Autodesk Inventor part; units mm, degrees
ref_plane "YZ Plane" through (0, 0, 0) normal (1, 0, 0) x (0, 1, 0)
ref_plane "XZ Plane" through (0, 0, 0) normal (0, 1, 0) x (-1, 0, 0)
ref_plane "XY Plane" through (0, 0, 0) normal (0, 0, 1) x (1, 0, 0)
sketch "Sketch1" plane through (0, 0, 0) normal (0, 1, 0) x (-1, 0, 0)
  line L0 (-40, -47.5) -> (40, -47.5)
  line L1 (40, -47.5) -> (40, 47.5)
  line L2 (40, 47.5) -> (-40, 47.5)
  line L3 (-40, 47.5) -> (-40, -47.5)
  line L4 (-40, -47.5) -> (40, 47.5) construction
  line L5 (40, -47.5) -> (-40, 47.5) construction
  line L6 (0, 0) -> (0, -31.5)
  line L7 (0, -31.5) -> (8.5, -31.5)
  line L8 (0, 0) -> (2.25, 0)
  line L9 (0, 0) -> (0, 17.5)
  line L10 (0, 17.5) -> (0, 19)
  line L11 (0, 19) -> (24, 19)
  line L12 (0, -17.5) -> (0, -19)
  line L13 (0, 31.5) -> (-19.5, 31.5)
  line L14 (0, 0) -> (0, 31.5)
  line L15 (0, 31.5) -> (8.5, 31.5)
  circle A0 centre (8.5, 31.5) radius 2.5
  line L16 (0, -19) -> (24, -19)
  circle A1 centre (24, -19) radius 2.5
  line L17 (0, 0) -> (0, -17.5)
  circle A2 centre (-19.5, 31.5) radius 2.5
  circle A3 centre (-19.5, 31.5) radius 2.5
  point P0 (0.5, 0.75)
  point P1 (0.5, -0.75)
  dimension "d0" = 80
  dimension "d1" = 95
  dimension "d2" = 17.5
  dimension "d3" = 8.5
  dimension "d5" = 31.5
  dimension "d6" = 24
  dimension "d7" = 2.25
  dimension "d12" = 19.5
extrude "Extrusion1" add sketch "Sketch1" along normal blind 10
sketch "Sketch2" plane through (0, 10, 0) normal (0, 1, 0) x (1, 0, 0)
  line L0 (-40, -47.5) -> (40, -47.5)
  line L1 (-40, -47.5) -> (-40, -36.5)
  line L2 (-40, 47.5) -> (-40, -47.5)
  line L3 (-40, -36.5) -> (-33.6491, -47.5)
  line L4 (-40, -36.5) -> (-27.2983, -36.5) construction
  line L5 (-33.6491, -47.5) -> (-33.6491, -43.5)
  line L6 (-40, -36.5) -> (-40, -33.5)
  line L7 (-33.6491, -47.5) -> (-33.6491, -45.5)
  line L8 (-32.6491, -47.5) -> (-31.6491, -47.5)
  line L9 (0, 0) -> (0, -47.5)
  line L10 (-40, -33.5) -> (-31, -33.5)
  line L11 (-31, -33.5) -> (-31, -47.5)
  line L12 (-33.6491, -47.5) -> (-31, -47.5)
  line L13 (40, -47.5) -> (40, -36.5)
  line L14 (40, -36.5) -> (33.6491, -47.5)
  line L15 (40, -36.5) -> (27.2983, -36.5) construction
  line L16 (33.6491, -47.5) -> (33.6491, -43.5)
  line L17 (40, -36.5) -> (40, -33.5)
  line L18 (33.6491, -47.5) -> (33.6491, -45.5)
  line L19 (32.6491, -47.5) -> (31.6491, -47.5)
  line L20 (40, -33.5) -> (31, -33.5)
  line L21 (31, -33.5) -> (31, -47.5)
  line L22 (33.6491, -47.5) -> (31, -47.5)
  line L23 (-40, 47.5) -> (-31, 47.5)
  line L24 (-31, 47.5) -> (-31, 33.5)
  line L25 (-31, 33.5) -> (-40, 33.5)
  line L26 (-40, 33.5) -> (-40, 47.5)
  line L27 (40, -47.5) -> (40, 47.5)
  line L28 (40, 47.5) -> (31, 47.5)
  line L29 (31, 47.5) -> (31, 33.5)
  line L30 (31, 33.5) -> (40, 33.5)
  line L31 (40, 33.5) -> (40, 47.5)
  dimension "d15" = 11
  dimension "d16" = 60
  dimension "d18" = 3
  dimension "d20" = 2
  dimension "d21" = 9
  dimension "d22" = 9
  dimension "d23" = 14
  dimension "d24" = 9
  dimension "d25" = 14
extrude "Extrusion2" add sketch "Sketch2" along normal blind 100 contours L2 L23 L24 L25 | L30 L29 L28 L27 | L21 L20 L17 L14 L0 | L3 L2 L10 L11 L0
sketch "Sketch4" plane through (0, 110, 0) normal (0, 1, 0) x (1, 0, 0)
  line L0 (-40, 47.5) -> (-40, 33.5)
  line L1 (-40, 33.5) -> (-31, 33.5)
  line L2 (-31, 33.5) -> (-31, 47.5)
  line L3 (-31, 47.5) -> (-40, 47.5)
  line L4 (40, 47.5) -> (31, 47.5)
  line L5 (31, 47.5) -> (31, 33.5)
  line L6 (31, 33.5) -> (40, 33.5)
  line L7 (40, 33.5) -> (40, 47.5)
  line L8 (33.6491, -47.5) -> (40, -36.5)
  line L9 (40, -36.5) -> (40, -33.5)
  line L10 (40, -33.5) -> (31, -33.5)
  line L11 (31, -33.5) -> (31, -47.5)
  line L12 (31, -47.5) -> (33.6491, -47.5)
  line L13 (-31, -47.5) -> (-31, -33.5)
  line L14 (-33.6491, -47.5) -> (-31, -47.5)
  line L15 (-31, -47.5) -> (-31, -33.5)
  line L16 (-31, -33.5) -> (-40, -33.5)
  line L17 (-40, -33.5) -> (-40, -36.5)
  line L18 (-40, -36.5) -> (-33.6491, -47.5)
  line L19 (-33.6491, -47.5) -> (-40, -36.5)
  line L20 (-40, -36.5) -> (-40, -47.5)
  line L21 (-40, -47.5) -> (-33.6491, -47.5)
  line L22 (40, -36.5) -> (33.6491, -47.5)
  line L23 (33.6491, -47.5) -> (40, -47.5)
  line L24 (40, -47.5) -> (40, -36.5)
  line L25 (-40, 47.5) -> (40, 47.5)
  line L26 (-40, 47.5) -> (-40, -47.5)
  line L27 (40, -47.5) -> (-40, -47.5)
  line L28 (-40, -47.5) -> (40, -47.5)
  line L29 (40, -47.5) -> (40, 47.5)
  line L30 (31, 33.5) -> (31, 47.5)
  line L31 (31, 47.5) -> (40, 47.5)
  line L32 (31, 47.5) -> (31, -33.5)
  line L33 (40, -33.5) -> (31, -33.5)
  line L34 (-40, -33.5) -> (-31, -33.5)
  line L35 (31, -33.5) -> (-31, -33.5)
  line L36 (-31, -33.5) -> (-31, 47.5)
  line L37 (-31, 47.5) -> (-31, 33.5)
  line L38 (-40, 47.5) -> (-31, 47.5)
  line L39 (-31, 47.1909) -> (-31, 33.5)
  line L40 (-40, 47.5) -> (-40, 33.5)
  line L41 (-31, 33.5) -> (-40, 33.5)
  line L42 (31, 33.5) -> (40, 33.5)
  line L43 (31, 33.5) -> (40, 33.5)
  point P0 (0, 0)
extrude "Extrusion3" add sketch "Sketch4" along normal blind 10 contours L3 L2 L1 L0 | L1 L36 L16 L26 | L16 L13 L14 L18 L17 | L4 L7 L6 L5 | L35 L11 L27 L13 | L18 L21 L20 | L6 L29 L10 L32 | L10 L9 L8 L12 L11 | L8 L24 L23
sketch "Sketch5" plane through (40, 0, -47.5) normal (0, 0, -1) x (-1, 0, 0)
  line L0 (80, 0) -> (0, 0)
  line L1 (80, 0) -> (80, 120)
  line L2 (71, 120) -> (80, 120)
  line L3 (71, 10) -> (71, 120)
  line L4 (9, 10) -> (71, 10)
  line L5 (9, 10) -> (9, 120)
  line L6 (0, 120) -> (9, 120)
  line L7 (0, 0) -> (0, 120)
  line L8 (9, 110) -> (71, 110)
  line L9 (71, 110) -> (71, 120)
  line L10 (9, 120) -> (71, 120)
  line L11 (9, 110) -> (9, 120)
  line L12 (9, 110) -> (9, 113)
  line L13 (9, 10) -> (9, 120)
  line L14 (9, 113) -> (4.5, 113)
  line L15 (4.5, 113) -> (4.5, 117)
  line L16 (4.5, 117) -> (9, 117)
  line L17 (9, 117) -> (9, 113)
  line L18 (9, 117) -> (9, 113)
  line L19 (9, 113) -> (71, 113)
  line L20 (71, 10) -> (71, 120)
  line L21 (71, 113) -> (75.5, 113)
  line L22 (75.5, 113) -> (75.5, 117)
  line L23 (75.5, 117) -> (71, 117)
  line L24 (71, 113) -> (71, 117)
  line L25 (71, 113) -> (71, 117)
  line L26 (8.545, 117) -> (71, 117)
  point P0 (40, 0)
  dimension "d30" = 3
  dimension "d31" = 4
  dimension "d32" = 4
extrude "Extrusion4" cut sketch "Sketch5" against normal blind 88 contours L23 L22 L21 L3 | L3 L19 L5 L26 | L5 L14 L15 L16
sketch "Sketch6" plane through (0, 0, 0) normal (0, -1, 0) x (1, 0, 0)
  point P0 (0, 0)
Geometry check sheet. Reference: the model listing, model coordinates, mm. A direction names the side the tool comes from. Coordinates: 2 decimals unless noted, no trailing zeros. Loops run counter-clockwise (first coordinate to the right, second up) from the corner with the lowest first, then second, coordinate; pieces in that order, holes last.
Item 1: Sectioned sample at A-A, the plane z = 1.5. Record the boundary of the cut face in (x, y).
Item 2: Sectioned sample at B-B, the plane y = 28.5. Record the boundary of the cut face in (x, z).
Item 3: Go/stop test with flat-tipped pins: pin 1 Ø7 at (x, z) = (-8, 43) entering from -Y; pin 2 Ø1 at (x, z) = (9.5, -32.5) entering from +Y; pin 3 Ø1.5 at (x, y) = (-3, 119) entering from -Z. Record where each tip stops, or that it passes through.
Item 4: Release check for a two-part mould opening along X. For faces 5 (the face through (1, 0, 1)), 6 (the face through (-8.17, 4.93, 29.02)), 7 (the face through (0, 113, 35)), 8 (the face through (36.87, 59.3, 41.92)) record: released by +X, released by -X, zero draft, split by the parting line, or undercut.
Item 5: Access from +Z, -Z, +X, -X, +Y, -Y to the whole of each face (thin tool, end or side, straight path). Record for faces 1 (the face through (0, 110, 40)), 2 (the face through (36, 59, 33.5)), 3 (the face through (0, 118, 33.5)), 4 (the face through (-36.87, 59.3, 41.92)).
Item 6: Thickness scan on line 1 (Y direction, x = 14.5, z = 37); line 2 (Z direction, x = -32, y = 38.5); line 3 (X direction, y = 2, z = 31). Record the ranges inside material, lowest first.
Item 7: Sectioned sample at C-C, the plane x = 24. Record the boundary of the cut face in (y, z), then the cut area to 3 significant figures.
Item 8: Sectioned sample at D-D, the plane x = -8.5. Record the boundary of the cut face in (y, z), then the cut area to 3 significant figures.
Check result:
1. outline: (-40, 0) - (40, 0) - (40, 10) - (-40, 10) - close; (-40, 110) - (-31, 110) - (-31, 113) - (-35.5, 113) - (-35.5, 117) - (-31, 117) - (-31, 120) - (-40, 120) - close; (31, 110) - (40, 110) - (40, 120) - (31, 120) - (31, 117) - (35.5, 117) - (35.5, 113) - (31, 113) - close
2. outline: (-40, -47.5) - (-31, -47.5) - (-31, -33.5) - (-40, -33.5) - close; (-40, 33.5) - (-31, 33.5) - (-31, 47.5) - (-33.65, 47.5) - (-40, 36.5) - close; (31, -47.5) - (40, -47.5) - (40, -33.5) - (31, -33.5) - close; (31, 33.5) - (40, 33.5) - (40, 36.5) - (33.65, 47.5) - (31, 47.5) - close
3. pin 1: stops at y = 0
3. pin 2: stops at y = 10
3. pin 3: stops at z = 33.5
4. face 5: zero draft
4. face 6: undercut
4. face 7: undercut
4. face 8: released by +X
5. face 1: +Z, -Z
5. face 2: +X, -X
5. face 3: -Z, +Y
5. face 4: +Z, -X
6. line 1: y = 0 to 10, 110 to 113, 117 to 120
6. line 2: z = -47.5 to -33.5, 33.5 to 47.5
6. line 3: x = -40 to -10.95, -6.05 to 17.05, 21.95 to 40
7. outline: (0, -47.5) - (10, -47.5) - (10, 47.5) - (0, 47.5) - close; (110, 33.5) - (113, 33.5) - (113, 40.5) - (117, 40.5) - (117, 33.5) - (120, 33.5) - (120, 47.5) - (110, 47.5) - close
7. area: 1,060 mm2
8. outline: (0, -47.5) - (10, -47.5) - (10, 29) - (0, 29) - close; (0, 34) - (10, 34) - (10, 47.5) - (0, 47.5) - close; (110, 33.5) - (113, 33.5) - (113, 40.5) - (117, 40.5) - (117, 33.5) - (120, 33.5) - (120, 47.5) - (110, 47.5) - close
8. area: 1,010 mm2
